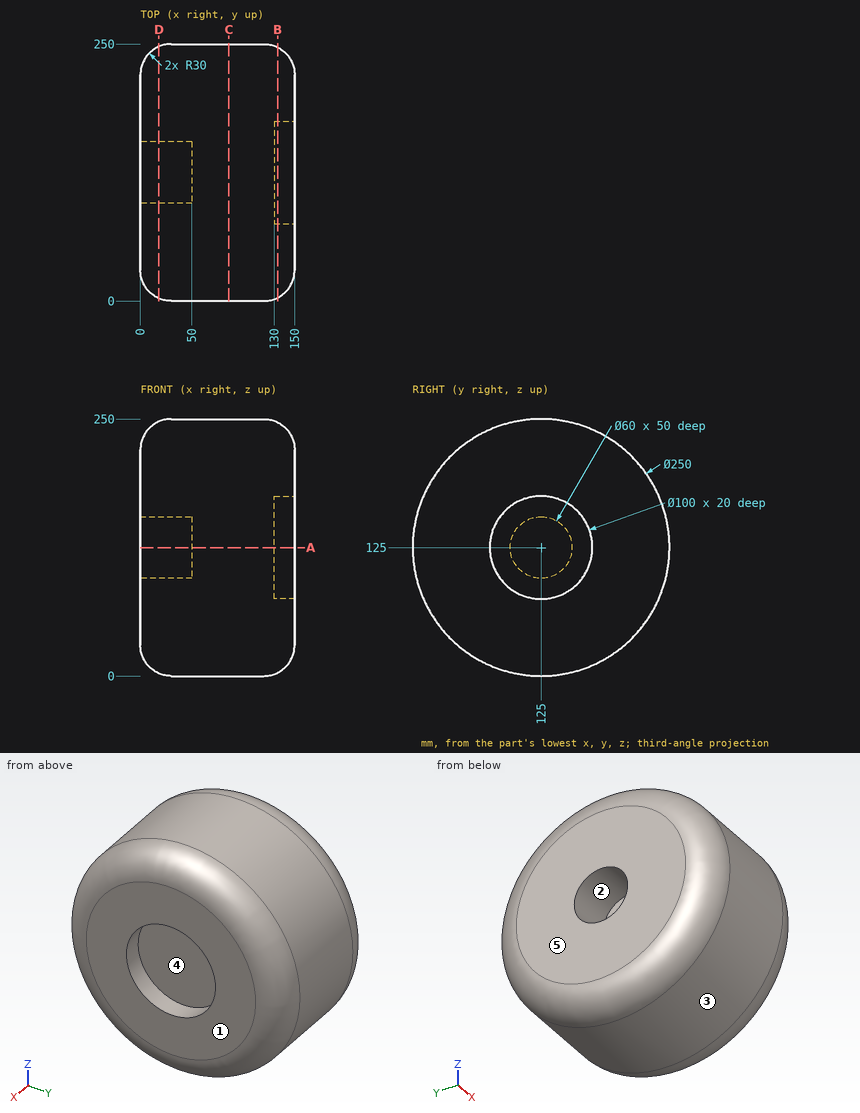
Verification items for this drawing (mm, ordinates from the low corner). A direction names the side the tool comes from. Coordinates: 2 decimals unless noted, no trailing zeros. Write each loop counter-clockwise with the first axis right and the second up, starting at its lowest first coordinate (ties: lowest second). Pieces come first, ordered by that corner, then holes. Notation, with made-up numbers: (53.5, 65) -> (58.5, 65) arc R22 cw to (58.5, 81) -> close; hole circle Ø9 at (41, 30). An arc over 180 degrees is marked (long way). Use CSV: the item, a comma, the result in double quotes. Start each with the question number.
Item 1: Mould release check, pull along Y, two halves, no side actions. Record for the marked faces 1, 2 and 3: released by +Y, released by -Y, zero draft, split by the parting line, or undercut.
Item 2: Cross-section at B-B, the plane x = 133.5. Record the cut outline in (y, z), plus the area to 3 significant figures.
Item 3: Cross-section at A-A, the plane z = 125. Record the cut outline in (x, y).
Item 4: Cross-section at D-D, the plane x = 18. Record the cut outline in (y, z), plus the area to 3 significant figures.
Item 5: Thickness scan on line 1 (Y direction, x = 18, z = 125); line 2 (Y direction, x = 134.5, z = 125); line 3 (Z direction, x = 79.5, y = 177.5). Record the ranges inside material, lowest first.
Item 6: Set-up check for the marked faces 4 and 5: record each of +Z, -Z, +X, -X, +Y, -Y from which the full face is reachable in a straight line by a thin tool's end or side.
Item 7: Cross-section at C-C, the plane x = 86. Record the cut outline in (y, z), plus the area to 3 significant figures.
Item 8: Depth check by flat-ended pin: pin 1 Ø1.5 at (x, y) = (95.5, 155.5) entering from +Z; pin 2 Ø10 at (x, y) = (63, 156) entering from -Z; pin 3 Ø8 at (x, y) = (51.5, 162) entering from -Z. Enter the tip coordinate at first touch or a pass-through.
Answers:
1,face 1,"zero draft"
1,face 2,"undercut"
1,face 3,"split by the parting line"
2,outline,"circle Ø243.58 at (125, 125); hole circle Ø100 at (125, 125)"
2,area,"38,700 mm^2"
3,outline,"(0, 30) arc R30 ccw to (30, 0) -> (120, 0) arc R30 ccw to (150, 30) -> (150, 75) -> (130, 75) -> (130, 175) -> (150, 175) -> (150, 220) arc R30 ccw to (120, 250) -> (30, 250) arc R30 ccw to (0, 220) -> (0, 155) -> (50, 155) -> (50, 95) -> (0, 95) -> close"
4,outline,"circle Ø244.99 at (125, 125); hole circle Ø60 at (125, 125)"
4,area,"44,300 mm^2"
5,line 1,"2.5 to 95, 155 to 247.5"
5,line 2,"3.74 to 75, 175 to 246.26"
5,line 3,"11.56 to 238.44"
6,face 4,"+X"
6,face 5,"+Z, -Z, -X, +Y, -Y"
7,outline,"circle Ø250 at (125, 125)"
7,area,"49,100 mm^2"
8,pin 1,"z = 246.41"
8,pin 2,"z = 2.73"
8,pin 3,"z = 4.43"
